The listing builds one solid part. Answer for the finished solid, in the listing's coordinates (mm). A direction names the side the tool comes from. Give positions to 0.01 mm unless a question says otherwise; leave off trailing zeros. Write each loop counter-clockwise with the first axis right and the second up, starting at its lowest first coordinate (ties: lowest second). Pieces come first, ordered by that corner, then holes.
Autodesk Inventor part; units mm, degrees
ref_plane "YZ Plane" through (0, 0, 0) normal (1, 0, 0) x (0, 1, 0)
ref_plane "XZ Plane" through (0, 0, 0) normal (0, 1, 0) x (-1, 0, 0)
ref_plane "XY Plane" through (0, 0, 0) normal (0, 0, 1) x (1, 0, 0)
sketch "Sketch2" plane through (0, 0, 0) normal (1, 0, 0) x (0, 1, 0)
  line L0 (0, 8.1606) -> (0, -1.3601)
  line L1 (-18.1996, 0) -> (16.4587, 0) construction
  arc A0 (-12.1735, 6.8) -> (-12.1757, 2.2019) centre (-10.2473, 4.5) ccw
  arc A1 (10.4508, 1.0716) -> (9.6493, 5.6) centre (8.1527, 3) ccw
  circle A2 centre (8.1527, 3) radius 1.3
  circle A3 centre (-10.2473, 4.5) radius 1.3
  line L2 (-0.3473, 3) -> (-5.3473, 3)
  line L3 (-9.5516, 0) -> (-12.1757, 2.2019)
  line L4 (9.5516, 0) -> (10.4508, 1.0716)
  line L5 (-9.5516, 0) -> (9.5516, 0)
  line L6 (-9.876, 6.8) -> (-5.3473, 3)
  line L7 (9.6493, 5.6) -> (6.7961, 5.6)
  line L8 (6.7961, 5.6) -> (-0.3473, 3)
  line L9 (-12.1735, 6.8) -> (-9.876, 6.8)
  point P0 (0, 0)
  dimension "d6" = 3
  dimension "d7" = 3
  dimension "d9" = 4.5
  dimension "d10" = 18.4
  dimension "d16" = 3
  dimension "d17" = 2.6
  dimension "d36" = 40
  dimension "d37" = 6.8
  dimension "d38" = 5.6
  dimension "d39" = 8.5
  dimension "d40" = 5
  dimension "d41" = 3
  dimension "d42" = 160
  dimension "d43" = 40
extrude "Extrusion1" add sketch "Sketch2" along normal mid plane 12
shell "Shell1" thickness 1 removed faces 11 at (2, -12.3599, 2.37) at (2, 9.8602, 5.4667) at (2, 9.4358, 2.7915) at (2, -8.9642, 4.2915) at (2, -3.6807, 3) at (-2, -11.301, 1.4679) at (2, 10.1511, 0.7144) at (2, 2.0338, 3.8667) at (2, 7.7472, 5.6) at (-2, -6.8569, 4.2667) at (-2, -10.6418, 6.8)
fillet "Fillet2" radius 0.5 2 edges at (-5, -0.1763, 1) (5, -0.1763, 1)
fillet "Fillet3" radius 1 2 edges at (6, 0, 0) (-6, 0, 0)
sketch "Sketch5" plane through (6, -9.5516, 0) normal (0, 0, -1) x (-1, 0, 0)
  line L0 (1, 17.3423) -> (2, 17.3423)
  line L1 (10, 17.3423) -> (11, 17.3423)
  arc A0 (2, 17.3423) -> (4, 19.3423) centre (2, 19.3423) ccw
  arc A1 (8, 19.3423) -> (10, 17.3423) centre (10, 19.3423) ccw
  line L2 (4, 19.3423) -> (4, 20.5415)
  line L3 (4, 20.5415) -> (1, 20.5415)
  line L4 (8, 19.3423) -> (8, 20.5415)
  line L5 (8, 20.5415) -> (11, 20.5415)
  line L6 (1, 20.5415) -> (1, 17.3423)
  line L7 (11, 20.5415) -> (11, 17.3423)
  line L8 (1, -1.7876) -> (1, 20.3024)
  line L9 (11, 20.3024) -> (11, -1.7876)
  line L10 (10.5, 19.9423) -> (1.5, 19.9423)
  point P0 (6, -9.8516)
  dimension "d47" = 2
  dimension "d53" = 3.1991
  dimension "d54" = 3
  dimension "d55" = 3.1991
  dimension "d56" = 3
  dimension "d57" = 2
  dimension "d58" = 2.6
extrude "Extrusion4" cut sketch "Sketch5" against normal up to next
sketch "Sketch7" plane through (-4.5, -10.7434, 1) normal (0, 0, 1) x (1, 0, 0)
  line L0 (6.5, 20.5341) -> (6.5, 21.1341)
  line L1 (2.5, 21.1341) -> (6.5, 21.1341)
  line L2 (-0.5, 1.1918) -> (11.5, 1.1918)
  line L3 (6.5, 20.295) -> (2.5, 20.295)
  line L4 (-0.5, 1.1918) -> (9.5, 1.1918)
  line L5 (9.5, 1.1918) -> (9.5, -0.8082)
  line L6 (9.5, -0.8082) -> (-0.5, -0.8082)
  line L7 (-0.5, -0.8082) -> (-0.5, 1.1918)
  line L8 (-0.5, -1.4301) -> (-0.5, 0.8674)
  line L9 (2.5, 21.1341) -> (6.5, 21.1341)
  line L10 (6.5, 21.1341) -> (6.5, 20.5341)
  line L11 (6.5, 20.5341) -> (2.5, 20.5341)
  line L12 (2.5, 20.5341) -> (2.5, 21.1341)
  point P0 (2.5, 20.5341)
  point P1 (4.5, 10.7434)
  point P2 (9.5, -0.5959)
  dimension "d52" = 2
extrude "Extrusion5" cut sketch "Sketch7" along normal through all both and the other way through all
sketch "Sketch8" plane through (0, 0, 0) normal (1, 0, 0) x (0, 1, 0)
  line L0 (-9.5516, 1) -> (7.7907, 1)
  line L1 (-9.5516, 0) -> (9.5516, 0)
  line L2 (-12.0753, 1.6595) -> (-11.4325, 2.4256)
  line L3 (-9.5516, 1) -> (-9.5516, 0)
  line L4 (-11.4325, 2.4256) -> (-9.873, 1.117)
  arc A0 (-9.873, 1.117) -> (-9.5516, 1) centre (-9.5516, 1.5) ccw
  line L5 (-12.0753, 1.6595) -> (-10.5158, 0.3509)
  arc A1 (-10.5158, 0.3509) -> (-9.5516, 0) centre (-9.5516, 1.5) ccw
  point P0 (0, 0)
  dimension "d61" = 50
  dimension "d62" = 1
  dimension "d63" = 1.5
  dimension "d64" = 3
extrude "Extrusion6" add sketch "Sketch8" along normal mid plane 8
properties material "Steel"
Item 1: Each of these flat-tipped pins is pushed along its axis until it touches: P1, Ø6, axis at x = 1, y = -4, coming from the +Z side; P2, Ø3.5, axis at y = 8.15, z = 3, coming from the -X side; P3, Ø1.6, axis at y = -10.25, z = 4.5, coming from the -X side; P4, Ø7, axis at x = -2, y = -3, coming from the +Z side. Where does it stop, or does it pass through?
Conclusion:
P1: stops at z = 1
P2: stops at x = -6
P3: passes through
P4: stops at z = 3
Item 2: A cutting plane is placed at B-B, the plane x = -0.75. Give the vertices of the cut face in (y, z), plus the area to 3 significant figures.
Conclusion:
outline: (-12.08, 1.66) - (-10.52, 0.35) arc R1.5 ccw to (-9.55, 0) - (9.55, 0) - (9.79, 0.28) - (9.79, 1) - (-9.55, 1) arc R0.5 cw to (-9.87, 1.12) - (-11.43, 2.43) - close
area: 22.0 mm2
Item 3: A cutting plane is placed at C-C, the plane y = -3. Give the vertices of the cut face in (x, z).
Conclusion:
outline: (-6, 1) arc R1 ccw to (-5, 0) - (5, 0) arc R1 ccw to (6, 1) - (6, 3) - (5, 3) - (5, 1.5) arc R0.5 cw to (4.5, 1) - (-4.5, 1) arc R0.5 cw to (-5, 1.5) - (-5, 3) - (-6, 3) - close
Item 4: Determine the mould class of faces 5 (the face through (5.493, -13.247, 4.465)), 6 (the face through (-2.57, 8.39, 0.49)), 7 (the face through (5.493, -7.643, 4.927)) for opening direction Y: pulls with the +Y half, pulls with the -Y half, needs draft (parallel to the pull), parting line crosses it, or undercut.
Conclusion:
face 5: pulls with the -Y half
face 6: pulls with the +Y half
face 7: undercut
Item 5: Consider probe 1 along X at (y, z) = (6.5, 1.75); probe 2 along Z at (x, y) = (3, 7); probe 3 along X at (y, z) = (8.5, 0.5). Determine where each line is inside the solid, lowest interval first.
Conclusion:
probe 1: x = -6 to -5, 5 to 6
probe 2: z = 0 to 1
probe 3: x = -5.87 to -5, -2.47 to 2.47, 5 to 5.87
Item 6: A cutting plane is placed at A-A, the plane z = 5. Give the vertices of the cut face in (x, y), plus the area to 3 significant figures.
Conclusion:
outline: (-6, -13.21) - (-5, -13.21) - (-5, -11.45) - (-6, -11.45) - close; (-6, -9.05) - (-5, -9.05) - (-5, -7.73) - (-6, -7.73) - close; (-6, 5.15) - (-5, 5.15) - (-5, 10.39) - (-6, 10.39) - close; (5, -13.21) - (6, -13.21) - (6, -11.45) - (5, -11.45) - close; (5, -9.05) - (6, -9.05) - (6, -7.73) - (5, -7.73) - close; (5, 5.15) - (6, 5.15) - (6, 10.39) - (5, 10.39) - close
area: 16.6 mm2
Item 7: Which of the six approach directions +Z, -Z, +X, -X, +Y, -Y give full straight-line access (tool end or side, diameter ignored) to faces 1 (the face through (5.5, -11, 6.8)), 2 (the face through (4.5, -9.552, 0.6)), 3 (the face through (5.49, -10.85, 1.09)), 4 (the face through (-5.5, -2.8, 3))?
Conclusion:
face 1: +Z, +X, -X, +Y, -Y
face 2: +Z, -Z, -Y
face 3: -Z, +X, -Y
face 4: +Z, +X, -X
Item 8: A cutting plane is placed at D-D, the plane x = 3.75. Give the vertices of the cut face in (y, z), plus the area to 3 significant figures.
Conclusion:
outline: (-12.08, 1.66) - (-10.52, 0.35) arc R1.5 ccw to (-9.55, 0) - (7.81, 0) - (7.81, 1) - (-9.55, 1) arc R0.5 cw to (-9.87, 1.12) - (-11.43, 2.43) - close
area: 20.1 mm2
